Build history of the part. All positions in model axes, mm. A direction names the side the tool comes from. Coordinates: 2 decimals unless noted, no trailing zeros. Write each loop counter-clockwise with the first axis right and the second up, starting at its lowest first coordinate (ties: lowest second). Pieces come first, ordered by that corner, then holes.
```python
from build123d import *

# Parameters (mm, degrees)
BOSS_EXTRUDE1_DEPTH = 150
SKETCH1_3_W         = 350
SKETCH1_3_H         = 240
BOSS_EXTRUDE2_DEPTH = 10


with BuildPart() as part:
    # Sketch1 → Boss-Extrude1 (new body)
    with BuildSketch(Plane(origin=(0, 0, 0), x_dir=(1, 0, 0), z_dir=(0, 1, 0))):
        Polygon((175, 120), (175, -120), (195, -120), (195, 140), (-195, 140), (-195, -120), (-175, -120), (-175, 120), align=None)
    extrude(amount=BOSS_EXTRUDE1_DEPTH)

    # Sketch1_3 → Boss-Extrude2 (add)
    with BuildSketch(Plane(origin=(0, 0, 0), x_dir=(1, 0, 0), z_dir=(0, 1, 0))):
        Rectangle(SKETCH1_3_W, SKETCH1_3_H)
        Polygon((175, 120), (175, -120), (195, -120), (195, 140), (-195, 140), (-195, -120), (-175, -120), (-175, 120), align=None)
    extrude(amount=-BOSS_EXTRUDE2_DEPTH)


solid = part.part
```
1. Saw through at C-C on x = -73. List the corners of the cut face in (y, z).
Computed values:
outline: (-10, -140) - (150, -140) - (150, -120) - (0, -120) - (0, 120) - (-10, 120) - close
2. Saw through at A-A on y = 120.5. List the corners of the cut face in (x, z), plus the area to 3 significant figures.
Computed values:
outline: (-195, -140) - (195, -140) - (195, 120) - (175, 120) - (175, -120) - (-175, -120) - (-175, 120) - (-195, 120) - close
area: 17,400 mm2
3. Mould opens along X. For faces 3 (the face through (-2, 74, -120)), 4 (the face through (-3, -10, -12)), 5 (the face through (-195, 71, -12)) say: +X half, -X half, draft (parallel to the pull), parting line (faces both ways), or undercut.
Computed values:
face 3: undercut
face 4: draft
face 5: -X half
4. Saw through at B-B on z = 50.5. List the corners of the cut face in (x, y).
Computed values:
outline: (-195, -10) - (195, -10) - (195, 150) - (175, 150) - (175, 0) - (-175, 0) - (-175, 150) - (-195, 150) - close
5. Flat gauge pins, fed straight in: pin 1 (2 mm diameter, centred on x = -68, z = -45.5, fed in from +Y); pin 2 (4 mm diameter, centred on x = 87, y = 61, fed in from +Z). Where does each tip first touch, or does it go through?
Computed values:
pin 1: stops at y = 0
pin 2: stops at z = -120
6. 3-axis set-ups, long thin cutter, end or side, ignore diameter. For faces 1 (the face through (-1, -1, 120)), 2 (the face through (175, 74, -2)): which of +Z, -Z, +X, -X, +Y, -Y reach the whole face in a straight line?
Computed values:
face 1: +Z, +X, -X, +Y, -Y
face 2: +Z, +Y
7. Probe line 1 along X through (y, z) = (102, -60); line 2 along Z through (x, y) = (-19, 125); line 3 along Y through (x, z) = (105.5, -111). List the from-to ranges inside material, lowest first.
Computed values:
line 1: x = -195 to -175, 175 to 195
line 2: z = -140 to -120
line 3: y = -10 to 0
